Autodesk Inventor part; units mm, degrees
ref_plane "YZ Plane" through (0, 0, 0) normal (1, 0, 0) x (0, 1, 0)
ref_plane "XZ Plane" through (0, 0, 0) normal (0, 1, 0) x (-1, 0, 0)
ref_plane "XY Plane" through (0, 0, 0) normal (0, 0, 1) x (1, 0, 0)
sketch "Sketch1" plane through (0, 0, 0) normal (1, 0, 0) x (0, 1, 0)
  line L0 (0, 0) -> (55, 0)
  line L1 (55, 0) -> (55, 20)
  line L2 (55, 20) -> (0, 20)
  line L3 (0, 20) -> (0, 0)
  line L4 (55, 10) -> (0, 10) construction
  circle A0 centre (40, 10) radius 2.6
  circle A1 centre (15, 10) radius 2.6
  dimension "d0" = 55
  dimension "d1" = 20
  dimension "d2" = 5.2
  dimension "d3" = 5.2
  dimension "d4" = 15
  dimension "d5" = 15
extrude "Extrusion1" add sketch "Sketch1" along normal blind 5
sketch "Sketch2" plane through (0, 0, 20) normal (0, 0, 1) x (1, 0, 0)
  line L0 (0, 48.25) -> (29, 48.25)
  line L1 (29, 48.25) -> (29, 55)
  line L2 (29, 55) -> (0, 55)
  line L3 (0, 55) -> (0, 48.25)
  line L4 (0, 0) -> (29, 0)
  line L5 (29, 0) -> (29, 6.75)
  line L6 (29, 6.75) -> (0, 6.75)
  line L7 (0, 6.75) -> (0, 0)
  line L8 (0, 55) -> (5, 55)
  line L9 (0, 0) -> (0, 55)
  line L10 (0, 55) -> (0, 0)
  line L11 (0, 0) -> (5, 0)
  line L12 (5, 55) -> (5, 0)
  line L13 (0, 55) -> (5, 55)
  line L14 (29, 55) -> (24, 55)
  line L15 (24, 55) -> (24, 0)
  line L16 (24, 0) -> (29, 0)
  line L17 (29, 0) -> (29, 55)
  point P0 (5, 48.25)
  point P1 (5, 6.75)
  point P2 (24, 6.75)
  point P3 (24, 48.25)
  dimension "d8" = 29
  dimension "d9" = 29
  dimension "d12" = 6.75
  dimension "d13" = 41.5
  dimension "d33" = 5
extrude "Extrusion2" add sketch "Sketch2" along normal blind 23 contours L3 L2 L12 L0 | L12 L2 L15 L0 | L6 L12 L4 L7 | L6 L15 L4 L12
fillet "Fillet1" radius 12 4 edges at (24, 51.625, 43) (0, 51.625, 43) (24, 3.375, 43) (0, 3.375, 43)
sketch "Sketch3" plane through (0, 55, 0) normal (0, 1, 0) x (1, 0, 0)
  circle A0 centre (12, -31) radius 2.75
  arc A1 (0, -31) -> (24, -31) centre (12, -31) ccw
  point P0 (0, 0)
  dimension "d17" = 5.5
extrude "Extrusion3" cut sketch "Sketch3" against normal through all
sketch "Sketch4" plane through (0, 0, 0) normal (0, 0, -1) x (-1, 0, 0)
  line L0 (0, 55) -> (-5, 55)
  line L1 (0, 55) -> (-29, 55)
  line L2 (-29, 55) -> (-29, 51.75)
  line L3 (-29, 51.75) -> (0, 51.75)
  line L4 (0, 51.75) -> (0, 55)
  line L5 (0, 6.75) -> (0, 0)
  line L6 (-29, 0) -> (-29, 6.75)
  line L7 (0, 0) -> (-29, 0)
  line L8 (-29, 0) -> (-29, 3.25)
  line L9 (-29, 3.25) -> (0, 3.25)
  line L10 (0, 3.25) -> (0, 0)
  dimension "d26" = 3.25
  dimension "d27" = 3.25
extrude "Extrusion4" cut sketch "Sketch4" against normal through all
chamfer "Chamfer3" distance 2.5 angle 45 2 edges at (9.25, 48.25, 31) (9.25, 6.75, 31)
chamfer "Chamfer4" distance 20 distance2 19 1 edges at (5, 50, 20) measured on face at (5, 23.6407, 2.523)
chamfer "Chamfer5" distance 20 distance2 19 1 edges at (5, 5, 20) measured on face at (5, 22.474, 2.523)
equation "\"d3\" = d2"
equation "\"d5\" = d4"
equation "\"d9\" = d8"
properties part number "Y Axis Drag Chain Mount Bolted"
Geometry check sheet. Reference: the model listing, model coordinates, mm. A direction names the side the tool comes from. Round coordinates to 2 decimals unless told otherwise and drop trailing zeros. Order: outer loops, then holes, each group sorted by start corner. A loop starts at its lowest first (then second) coordinate and runs counter-clockwise, first axis right, second up. Notation, with made-up numbers: M 42,42.25 L 91,42.25 A7 ccw 91,55.25 Z; hole C 83,18 d10. An arc over 180 degrees is marked long. Answer in a Markdown table with one row per item. Add a question column.
Item 1: Draft check along X on faces 6 (the face through (13.34, 50.59, 28.42)), 7 (the face through (3.61, 4.98, 39.58)), 8 (the face through (20.58, 49.98, 39.39)). Enter one of: released by +X, released by -X, zero draft, split by the parting line, or undercut.
Item 2: Sectioned sample at A-A, the plane y = 40. Enter the section's corners in (x, z).
Item 3: Sectioned sample at C-C, the plane x = 2.75. Enter the section's corners in (y, z).
Item 4: Depth check by flat-ended pin: pin 1 Ø7 at (y, z) = (15, 10) entering from +X; pin 2 Ø4.5 at (x, z) = (12, 31) entering from -Y; pin 3 Ø12 at (x, y) = (20.5, 43) entering from -Z; pin 4 Ø4 at (x, y) = (1.5, 33) entering from +Z. Enter the tip coordinate at first touch or a pass-through.
Item 5: Sectioned sample at B-B, the plane z = 11. Enter the section's corners in (x, y), plus the area to 3 significant figures.
Item 6: Material ranges on L1, parallel to Y at x = 18, z = 33; L2, parallel to Z at x = 2.1, y = 40; L3, parallel to X at y = 3.6, z = 31, recorded low to high. Write a range as [from, to].
Item 7: Sectioned sample at D-D, the plane z = 37.5. Enter the section's corners in (x, y).
Item 8: Set-up check for faces 1 (the face through (13.34, 4.41, 33.58)), 2 (the face through (5, 27, 10)), 3 (the face through (2, 28, 20)), 4 (the face through (9.5, 6.75, 26)), 5 (the face through (2.5, 17.4, 11)): record each of +Z, -Z, +X, -X, +Y, -Y from which the full face is reachable in a straight line by a thin tool's end or side.
Filled in:
| question | item | result |
|---|---|---|
| 1 | face 6 | undercut |
| 1 | face 7 | released by -X |
| 1 | face 8 | released by +X |
| 2 | outline | M 0,0 L 5,0 L 5,7.4 L 0,7.4 Z; M 0,12.6 L 5,12.6 L 5,20 L 0,20 Z |
| 3 | outline | M 3.25,0 L 51.75,0 L 51.75,38.64 L 48.25,38.64 L 48.25,20 L 6.75,20 L 6.75,38.64 L 3.25,38.64 Z; hole C 15,10 d5.2; hole C 40,10 d5.2 |
| 4 | pin 1 | stops at x = 5 |
| 4 | pin 2 | passes through |
| 4 | pin 3 | stops at z = 13.26 |
| 4 | pin 4 | stops at z = 20 |
| 5 | outline | M 0,3.25 L 15.45,3.25 L 15.45,6.75 L 5,6.75 L 5,12.6 L 0,12.6 Z; M 0,17.4 L 5,17.4 L 5,37.6 L 0,37.6 Z; M 0,42.4 L 5,42.4 L 5,48.25 L 15.45,48.25 L 15.45,51.75 L 0,51.75 Z |
| 5 | area | 268 mm² |
| 6 | L1 | y = [3.25, 6.75], [48.25, 51.75] |
| 6 | L2 | z = [0, 7.4], [12.6, 20] |
| 6 | L3 | x = [0, 9.25], [14.75, 24] |
| 7 | outline | M 1.91,3.25 L 22.09,3.25 L 22.09,6.75 L 1.91,6.75 Z; M 1.91,48.25 L 22.09,48.25 L 22.09,51.75 L 1.91,51.75 Z |
| 8 | face 1 | none |
| 8 | face 2 | +Z, -Z, +X |
| 8 | face 3 | +Z, +X, -X |
| 8 | face 4 | +Z, +X |
| 8 | face 5 | +X, -X |
